Source: CAD feature listing. Evaluate the final solid. Frame: model axes, mm. A direction names the side the tool comes from. Coordinates: 2 decimals unless noted, no trailing zeros. Loops run counter-clockwise (first coordinate to the right, second up) from the corner with the lowest first, then second, coordinate; pieces in that order, holes last.
Item 1: Section query A-A, the plane y = 0. Return the cut outline in (x, z).
Item 2: Reachability of faces 1 (the flat face through (-7, 7, 25)), 2 (the cylindrical face through (3.35, 56.43, 2.46)) from +Z, -Z, +X, -X, +Y, -Y: full face, straight path, thin tool, end or side. Return the list, or none.
Item 3: Line query: probe 1 along Y at (x, z) = (0, 16); probe 2 along Z at (x, y) = (10.5, 18); probe 3 along X at (y, z) = (-6, 48). Output: solid intervals per line, ascending.
Item 4: Pull-direction query (X, two-part tool) for faces 3 (the cylindrical face through (-14.985, -0.66, 34.58)), 4 (the flat face through (13, -13, 5)), 5 (the cylindrical face through (42.757, -0.319, 2.465)); classes: +X half, -X half, draft (parallel to the pull), parting line (faces both ways), or undercut.
Item 5: Section query B-B, the plane y = 50. Return the cut outline in (x, z), then the cut area to 4 significant figures.
Item 6: Pin query (flat end, axial travel): pin 1 Ø4 at (x, y) = (-30, -35) entering from +Z; pin 2 Ø5 at (y, z) = (2.5, 16) entering from +X; pin 3 Ø1.5 at (x, z) = (-9.5, 10.5) entering from +Y; pin 4 Ø13 at (x, y) = (0, -50) entering from +Z. Return the tip coordinate at first contact, or that it passes through.
Autodesk Inventor part; units mm, degrees
ref_plane "YZ Plane" through (0, 0, 0) normal (1, 0, 0) x (0, 1, 0)
ref_plane "XZ Plane" through (0, 0, 0) normal (0, 1, 0) x (-1, 0, 0)
ref_plane "XY Plane" through (0, 0, 0) normal (0, 0, 1) x (1, 0, 0)
sketch "Sketch1" plane through (0, 0, 0) normal (0, 0, 1) x (1, 0, 0)
  circle A0 centre (0, 0) radius 50 construction
  circle A1 centre (0, 50) radius 7.25
  circle A2 centre (-50, 0) radius 7.25
  circle A3 centre (0, -50) radius 7.25
  circle A4 centre (50, 0) radius 7.25
  circle A5 centre (0, 0) radius 15 construction
  circle A6 centre (0, 0) radius 62.5
  circle A7 centre (0, 0) radius 9.5
  dimension "d0" = 100
  dimension "d1" = 14.5
  dimension "d4" = 360
  dimension "d6" = 30
  dimension "d7" = 125
  dimension "d8" = 19
extrude "Extrusion1" add sketch "Sketch1" along normal blind 5
sketch "Sketch2" plane through (0, 0, 5) normal (0, 0, 1) x (1, 0, 0)
  circle A0 centre (0, 0) radius 15
  circle A1 centre (0, 0) radius 9.5
  dimension "d11" = 30
extrude "Extrusion2" add sketch "Sketch2" along normal blind 60
sketch "Sketch3" plane through (0, 0, 65) normal (0, 0, 1) x (1, 0, 0)
  circle A0 centre (0, 0) radius 15
  circle A1 centre (0, 0) radius 9.5
  line L0 (6.7175, -6.7175) -> (-8.4853, 8.4853)
  line L1 (-8.4853, 8.4853) -> (-10.6066, 6.364)
  line L2 (-10.6066, 6.364) -> (-8.4951, 4.2525)
  line L3 (-8.4853, 8.4853) -> (-6.364, 10.6066)
  line L4 (-6.364, 10.6066) -> (-4.2525, 8.4951)
  dimension "d14" = 21.5
  dimension "d15" = 3
  dimension "d16" = 3
extrude "Extrusion3" cut sketch "Sketch3" against normal blind 40 contours A1 L0 L3 L4 | A1 L2 L1 L0
properties part number "wheelFlangeMotor"
Verdict:
1. outline: (-62.5, 0) - (-57.25, 0) - (-57.25, 5) - (-62.5, 5) - close; (-42.75, 0) - (-9.5, 0) - (-9.5, 65) - (-15, 65) - (-15, 5) - (-42.75, 5) - close; (9.5, 0) - (42.75, 0) - (42.75, 5) - (15, 5) - (15, 65) - (9.5, 65) - close; (57.25, 0) - (62.5, 0) - (62.5, 5) - (57.25, 5) - close
2. face 1: +Z
2. face 2: +Z, -Z
3. probe 1: y = -15 to -9.5, 9.5 to 15
3. probe 2: z = 0 to 5
3. probe 3: x = -13.75 to -7.37, 7.37 to 13.75
4. face 3: parting line
4. face 4: draft
4. face 5: undercut
5. outline: (-37.5, 0) - (-7.25, 0) - (-7.25, 5) - (-37.5, 5) - close; (7.25, 0) - (37.5, 0) - (37.5, 5) - (7.25, 5) - close
5. area: 302.5 mm2
6. pin 1: stops at z = 5
6. pin 2: stops at x = 15
6. pin 3: stops at y = 12.18
6. pin 4: passes through
